The listing builds one solid part. Answer for the finished solid, in the listing's coordinates (mm). A direction names the side the tool comes from. Coordinates: 2 decimals unless noted, no trailing zeros. Write each loop counter-clockwise with the first axis right and the second up, starting at its lowest first coordinate (ties: lowest second). Pieces come first, ordered by that corner, then holes.
from build123d import *

# Parameters (mm, degrees)
F1_DEPTH   = 5
F3_DEPTH   = 20
F7_D       = 4.2
F7_ON_F5_D = 4.2
F7_ON_F4_D = 4.2
F8_R       = 5


with BuildPart() as f1:
    # F0 (on Top) → F1 (new body)
    with BuildSketch(Plane.XY):
        with BuildLine():
            Line((0, -50), (0, 0))
            Line((0, 0), (0, 50))
            Line((0, 50), (-25, 50))
            ThreePointArc((-25, 50), (-35.2512626585, 25.2512626585), (-60, 15))
            Line((-60, 15), (-65, 15))
            Line((-65, 15), (-65, 0))
            Line((-65, 0), (-65, -15))
            Line((-65, -15), (-60, -15))
            ThreePointArc((-60, -15), (-35.2512626585, -25.2512626585), (-25, -50))
            Line((-25, -50), (0, -50))
        make_face()
    extrude(amount=F1_DEPTH)

    # F2 (on face) → F3 (join)
    with BuildSketch(Plane.XY.offset(5)):
        Polygon((-20, 50), (-25, 50), (-25, 15), (-65, 15), (-65, 10), (-25, 10), (-25, -10), (-65, -10), (-65, -15), (-25, -15), (-25, -50), (-20, -50), align=None)
    extrude(amount=F3_DEPTH)

    # F7 (through all)
    with Locations(Plane.XY.offset(5)):
        with Locations((-10, -37.5), (-10, 0), (-10, 37.5)):
            Hole(F7_D / 2)

    # F7 on F5 (through all)
    with Locations(Plane(origin=(-25, 0, 0), x_dir=(0, -1, 0), z_dir=(-1, 0, 0))):
        with Locations((37.5, 15), (-37.5, 15)):
            Hole(F7_ON_F5_D / 2)

    # F7 on F4 (through all)
    with Locations(Plane.XZ.offset(15)):
        with Locations((-55, 15), (-35, 15)):
            Hole(F7_ON_F4_D / 2)

    # F8
    f8_edges = [f1.edges().sort_by_distance(p)[0] for p in [
        (-65, -12.5, 25),
        (-65, 12.5, 25),
        (-22.5, 50, 25),
        (-22.5, -50, 25),
        (0, -50, 2.5),
        (0, 50, 2.5),
        (-25, -15, 15),
        (-25, 15, 15),
    ]]
    fillet(f8_edges, radius=F8_R)


solid = f1.part
Q1. The part is cut by section A-A, the plane x = -10. Write down the section's boundary in (y, z).
Answers below:
outline: (-50, 0) - (-39.6, 0) - (-39.6, 5) - (-50, 5) - close; (-35.4, 0) - (-2.1, 0) - (-2.1, 5) - (-35.4, 5) - close; (2.1, 0) - (35.4, 0) - (35.4, 5) - (2.1, 5) - close; (39.6, 0) - (50, 0) - (50, 5) - (39.6, 5) - close
Q2. Find the intervals of material crossed by probe 1 along Y at (x, z) = (-61, 16.5); probe 2 along X at (y, z) = (14.5, 15.25); probe 3 along Y at (x, z) = (-22, 13.5), in increasing order.
Answers below:
probe 1: y = -15 to -10, 10 to 15
probe 2: x = -65 to -57.09, -52.91 to -37.09, -32.91 to -20
probe 3: y = -50 to -38.97, -36.03 to 36.03, 38.97 to 50
Q3. Given pin 1 (10 mm diameter, centred on y = 4.5, z = 15, fed in from -X); pin 2 (10.5 mm diameter, centred on x = -37, y = -37.5, fed in from +Z); pin 3 (10 mm diameter, centred on x = -47, z = 4.5, fed in from -Y); pin 4 (6 mm diameter, centred on y = -6.5, z = 20, fed in from +X), each flat-ended and moving along its own axis, determine where each tip first touches the part or whether it passes through.
Answers below:
pin 1: stops at x = -25
pin 2: passes through
pin 3: stops at y = -19.98
pin 4: stops at x = -20
Q4. The part is cut by section B-B, the plane x = -21. Write down the section's boundary in (y, z), then the cut area to 3 significant figures.
Answers below:
outline: (-50, 0) - (50, 0) - (50, 20) arc R5 ccw to (45, 25) - (-45, 25) arc R5 ccw to (-50, 20) - close; hole circle Ø4.2 at (-37.5, 15); hole circle Ø4.2 at (37.5, 15)
area: 2,460 mm2
Q5. The part is cut by section D-D, the plane z = 10.25. Write down the section's boundary in (x, y), then the cut area to 3 significant figures.
Answers below:
outline: (-65, -15) - (-30, -15) arc R5 cw to (-25, -20) - (-25, -50) - (-20, -50) - (-20, 50) - (-25, 50) - (-25, 20) arc R5 cw to (-30, 15) - (-65, 15) - (-65, 10) - (-25, 10) - (-25, -10) - (-65, -10) - close
area: 911 mm2
Q6. Which of the six approach directions +Z, -Z, +X, -X, +Y, -Y give full straight-line access (tool end or side, diameter ignored) to faces 1 (the face through (-27, -16, 15)), 2 (the face through (-12.4, 0.7, 5)), 3 (the face through (-20, -50, 3)), 4 (the face through (-34, 24, 5)), 5 (the face through (-25, 0, 15))?
Answers below:
face 1: +Z, -X, -Y
face 2: +Z, +X, +Y, -Y
face 3: +Z, -Z, +X, -X, -Y
face 4: +Z, -X, +Y
face 5: +Z, -X
Q7. The part is cut by section C-C, the plane y = 37.5. Write down the section's boundary in (x, z).
Answers below:
outline: (-27.31, 0) - (-12.1, 0) - (-12.1, 5) - (-20, 5) - (-20, 12.9) - (-25, 12.9) - (-25, 5) - (-27.31, 5) - close; (-25, 17.1) - (-20, 17.1) - (-20, 25) - (-25, 25) - close; (-7.9, 0) - (0, 0) - (0, 5) - (-7.9, 5) - close
Q8. Determine the mould class of faces 6 (the face through (-32.9, 12.53, 15.09)), 7 (the face through (-63, -13, 24)), 8 (the face through (-65, 4, 3)) for opening direction Z: released by +Z, released by -Z, zero draft, split by the parting line, or undercut.
Answers below:
face 6: undercut
face 7: released by +Z
face 8: zero draft
